Model file for the job. Use its own axes, mm. A direction names the side the tool comes from. Give positions to 0.01 mm unless a question says otherwise; leave off trailing zeros. Order: outer loops, then holes, each group sorted by start corner. A loop starts at its lowest first (then second) coordinate and runs counter-clockwise, first axis right, second up. Notation, with made-up numbers: (15, -15) - (65, -15) arc R21 ccw to (65, 3) - close; hole circle Ø11 at (72.5, -19). An arc over 180 degrees is marked (long way). Use CSV: the item, a comma, the result in double quotes. Start each with the question number.
(1) Band-saw the part on B-B, the plane y = -38. Give the cut face in (x, z), then the cut area to 3 significant figures.
(2) Probe L1, parallel to Z at x = 25.5, y = -58.5; L2, parallel to X at y = 0, z = 4; L3, parallel to Y at x = 41, z = 5.5. List the from-to ranges inside material, lowest first.
(3) Tool access for faces 1 (the flat face through (15, 0, 1)), 2 (the flat face through (0, -32, 1)): list every direction of +Z, -Z, +X, -X, +Y, -Y with a clear straight run to the whole face (end or side of a thin tool).
(4) Band-saw the part on A-A, the plane x = 16. Give the cut face in (y, z), then the cut area to 3 significant figures.
(5) Band-saw the part on C-C, the plane x = 34.5. Give the cut face in (y, z).
(6) Drop flat-ended pins along their axis: pin 1 Ø1.4 at (x, z) = (8, 1) entering from +Y; pin 2 Ø1 at (x, z) = (32, 3) entering from -Y; pin 3 Ø10 at (x, y) = (20, -30.5) entering from +Z. Give the stop position or say it passes through.
from build123d import *

# Parameters (mm, degrees)
F0_W     = 61
F0_H     = 63
F1_DEPTH = 1.8
F3_DEPTH = 30.5


with BuildPart() as f1:
    # F0 (on Top) → F1 (new body)
    with BuildSketch(Plane.XY):
        with Locations((30.5, -31.5)):
            Rectangle(F0_W, F0_H)
    extrude(amount=F1_DEPTH)

    # F2 (on face) → F3 (join)
    with BuildSketch(Plane.YZ.offset(61)):
        with BuildLine():
            Line((0, 1.8), (0, 0))
            ThreePointArc((0, 0), (2.1213203436, 0.8786796564), (3, 3))
            ThreePointArc((3, 3), (-0.6129289311, 5.9367189388), (-2.749545417, 1.8))
            Line((-2.749545417, 1.8), (0, 1.8))
        make_face()
        with BuildLine():
            ThreePointArc((-2.749545417, 1.8), (-1.6431676725, 0.4900199204), (0, 0))
            Line((0, 0), (0, 1.8))
            Line((0, 1.8), (-2.749545417, 1.8))
        make_face()
    extrude(amount=-F3_DEPTH)


solid = f1.part
Answer block:
1,outline,"(0, 0) - (61, 0) - (61, 1.8) - (0, 1.8) - close"
1,area,"110 mm2"
2,L1,"z = 0 to 1.8"
2,L2,"x = 30.5 to 61"
2,L3,"y = -1.66 to 1.66"
3,face 1,"+Z, -Z, -X, +Y"
3,face 2,"+Z, -Z, -X, +Y, -Y"
4,outline,"(-63, 0) - (0, 0) - (0, 1.8) - (-63, 1.8) - close"
4,area,"113 mm2"
5,outline,"(-63, 0) - (0, 0) arc R3 ccw (long way) to (-2.75, 1.8) - (-63, 1.8) - close"
6,pin 1,"stops at y = 0"
6,pin 2,"stops at y = -3"
6,pin 3,"stops at z = 1.8"
